Read the model definition and answer for the solid it produces. Units are mm, in the model's axes. Give positions to 0.01 mm unless a question says otherwise; leave off trailing zeros. Loops run counter-clockwise (first coordinate to the right, second up) from the corner with the lowest first, then second, coordinate; pieces in that order, holes last. Notation, with made-up numbers: (22, -4.75) -> (35, -4.75) arc R22 ccw to (35, 28.25) -> close; hole circle Ø11 at (66.5, 85.25). An arc over 180 degrees is marked (long way). Write each question's results on one line, items separated by ' | '. Start each with the question number.
Item 1: Section C-C on z = 6.25 is taken. Write down the section's boundary in (x, y).
Item 2: Determine the mould class of faces 1 (the flat face through (-11.5, -5, 4)), 2 (the cylindrical face through (-1.73, -7.81, 3.94)), 3 (the cylindrical face through (-1.041, 34.932, 3.944)), 4 (the flat face through (-0.16, -32.42, 5.04)) for opening direction X: +X half, -X half, draft (parallel to the pull), parting line (faces both ways), or undercut.
Item 3: Find the intervals of material crossed by line 1 (Y direction, x = 0, z = 5); line 2 (Y direction, x = 0, z = 2.25); line 3 (X direction, y = -0.5, z = 5.5), in increasing order.
Item 4: Each of these flat-tipped pins is pushed along its axis until it touches: P1, Ø3, axis at x = 9, z = 5.5, coming from the +Y side; P2, Ø1.5, axis at x = 4.5, z = 7, coming from the -Y side. Where does it stop, or does it pass through?
Item 5: Section B-B on y = 0 is taken. Write down the section's boundary in (x, z).
Item 6: Section A-A on x = 0 is taken. Write down the section's boundary in (y, z).
Item 7: Section D-D on x = 4.5 is taken. Write down the section's boundary in (y, z), and give its area (3 significant figures).
```python
from build123d import *

# Parameters (mm, degrees)
F0_R     = 8
F1_DEPTH = 8
F3_DEPTH = 23.001


with BuildPart() as f1:
    # F0 (on Top) → F1 (new body)
    with BuildSketch(Plane.XY):
        with BuildLine():
            Line((-11.5, 27), (-11.5, -38.5))
            Line((-11.5, -38.5), (11.5, -38.5))
            Line((11.5, -38.5), (11.5, 27))
            ThreePointArc((11.5, 27), (0, 38.5), (-11.5, 27))
        make_face()
        Circle(F0_R, mode=Mode.SUBTRACT)
        with Locations((0, 27)):
            Circle(F0_R, mode=Mode.SUBTRACT)
    extrude(amount=F1_DEPTH)

    # F2 (on face) → F3 (cut, through all)
    with BuildSketch(Plane(origin=(-11.5, 0, 0), x_dir=(0, -1, 0), z_dir=(-1, 0, 0))):
        Polygon((26.5, 8), (38.5, 2), (38.5, 8), align=None)
    extrude(amount=-F3_DEPTH, mode=Mode.SUBTRACT)


solid = f1.part
```
Findings:
1) outline: (-11.5, -30) -> (11.5, -30) -> (11.5, 27) arc R11.5 ccw to (-11.5, 27) -> close; hole circle Ø16 at (0, 0); hole circle Ø16 at (0, 27)
2) face 1: -X half | face 2: undercut | face 3: undercut | face 4: draft
3) line 1: -32.5 to -8, 8 to 19, 35 to 38.5 | line 2: -38 to -8, 8 to 19, 35 to 38.5 | line 3: -11.5 to -7.98, 7.98 to 11.5
4) P1: y = 35.72 | P2: y = -30
5) outline: (-11.5, 0) -> (-8, 0) -> (-8, 8) -> (-11.5, 8) -> close; (8, 0) -> (11.5, 0) -> (11.5, 8) -> (8, 8) -> close
6) outline: (-38.5, 0) -> (-8, 0) -> (-8, 8) -> (-26.5, 8) -> (-38.5, 2) -> close; (8, 0) -> (19, 0) -> (19, 8) -> (8, 8) -> close; (35, 0) -> (38.5, 0) -> (38.5, 8) -> (35, 8) -> close
7) outline: (-38.5, 0) -> (-6.61, 0) -> (-6.61, 8) -> (-26.5, 8) -> (-38.5, 2) -> close; (6.61, 0) -> (20.39, 0) -> (20.39, 8) -> (6.61, 8) -> close; (33.61, 0) -> (37.58, 0) -> (37.58, 8) -> (33.61, 8) -> close | area: 361 mm2
